from build123d import *

# Parameters (mm, degrees)
BOSS_EXTRUDE1_DEPTH       = 7
F_5_0MM_DOWEL_HOLE1_D     = 5
F_5_0MM_DOWEL_HOLE1_DEPTH = 7
SKETCH4_W                 = 66
SKETCH4_H                 = 37.5
BOSS_EXTRUDE2_DEPTH       = 13
SKETCH5_W                 = 65.8
SKETCH5_H                 = 37.3
BOSS_EXTRUDE3_DEPTH       = 22
FILLET1_R                 = 3
FILLET2_R                 = 2


with BuildPart() as part:
    # Sketch1 → Boss-Extrude1 (new body)
    with BuildSketch(Plane(origin=(0, 0, 0), x_dir=(1, 0, 0), z_dir=(0, 1, 0))):
        with BuildLine():
            Line((-41.327503189, 4.721250532), (-33, 15))
            Line((-33, 15), (-33, 26.5))
            Line((-33, 26.5), (33, 26.5))
            Line((33, 26.5), (33, 15))
            Line((33, 15), (41.327503189, 4.721250532))
            ThreePointArc((41.327503189, 4.721250532), (43, 0), (41.327503189, -4.721250532))
            Line((41.327503189, -4.721250532), (33, -15))
            Line((33, -15), (33, -26.5))
            Line((33, -26.5), (-33, -26.5))
            Line((-33, -26.5), (-33, -15))
            Line((-33, -15), (-41.327503189, -4.721250532))
            ThreePointArc((-41.327503189, -4.721250532), (-43, 0), (-41.327503189, 4.721250532))
        make_face()
    extrude(amount=BOSS_EXTRUDE1_DEPTH)

    # Ø5.0mm Dowel Hole1
    with Locations(Plane(origin=(0, 7, 0), x_dir=(1, 0, 0), z_dir=(0, 1, 0))):
        with Locations((-38.5, 0), (38.5, 0)):
            Hole(F_5_0MM_DOWEL_HOLE1_D / 2, depth=F_5_0MM_DOWEL_HOLE1_DEPTH)

    # Sketch4 → Boss-Extrude2 (add)
    with BuildSketch(Plane(origin=(0, 7, 0), x_dir=(1, 0, 0), z_dir=(0, 1, 0))):
        Rectangle(SKETCH4_W, SKETCH4_H)
    extrude(amount=BOSS_EXTRUDE2_DEPTH)

    # Sketch5 → Boss-Extrude3 (add)
    with BuildSketch(Plane(origin=(0, 20, 0), x_dir=(1, 0, 0), z_dir=(0, 1, 0))):
        Rectangle(SKETCH5_W, SKETCH5_H)
    extrude(amount=BOSS_EXTRUDE3_DEPTH)

    # Fillet1
    fillet1_edges = [part.edges().sort_by_distance(p)[0] for p in [
        (-33, 3.5, -26.5),
        (33, 3.5, -26.5),
        (33, 3.5, 26.5),
        (-33, 3.5, 26.5),
        (33, 13.5, 18.75),
        (33, 13.5, -18.75),
        (-33, 13.5, -18.75),
        (-33, 13.5, 18.75),
        (32.9, 31, 18.65),
        (32.9, 31, -18.65),
        (-32.9, 31, -18.65),
        (-32.9, 31, 18.65),
    ]]
    fillet(fillet1_edges, radius=FILLET1_R)

    # Fillet2
    fillet2_edges = [part.edges().sort_by_distance(p)[0] for p in [
        (32.9, 42, 0),
        (0, 42, 18.65),
        (0, 42, -18.65),
        (-32.9, 42, 0),
        (-32.021320344, 42, 17.771320344),
        (-32.021320344, 42, -17.771320344),
        (32.021320344, 42, -17.771320344),
        (32.021320344, 42, 17.771320344),
    ]]
    fillet(fillet2_edges, radius=FILLET2_R)


solid = part.part
Check sheet for the modelled part. Datum: model origin and axes. Units: mm. A direction names the side the tool comes from. Give positions to 0.01 mm unless a question says otherwise; leave off trailing zeros. Loops run counter-clockwise (first coordinate to the right, second up) from the corner with the lowest first, then second, coordinate; pieces in that order, holes last. Notation, with made-up numbers: M 53.5,61 L 110.5,61 A15 ccw 110.5,66 Z; hole C -17,9.25 d11. An arc over 180 degrees is marked long. Use a Markdown table: item, result. Add a question column.
Q1. Sectioned sample at D-D, the plane x = 20. Record the cut outline in (y, z).
Q2. Sectioned sample at A-A, the plane z = 0. Record the cut outline in (x, y), then the cut area to 3 significant figures.
Q3. Tool access check on faces 1 (the cylindrical face through (-32.14, 13.59, -17.85)), 2 (the cylindrical face through (32.04, 30.14, -17.75)), 3 (the flat face through (35.8, 7, -0.2)), 4 (the flat face through (-33, 10, 0)), 5 (the flat face through (0, 13, 18.75)). Record the directions out of +Z, -Z, +X, -X, +Y, -Y that give a thin tool (end or side, any length) a straight path to the whole face; none if there is none.
Q4. Scan lines: line 1 along Z through (x, y) = (-15, 11); line 2 along Y through (x, z) = (-12.5, -20); line 3 along X through (y, z) = (27.5, 10.5). Record each from-to range of solid material in increasing order. Write a range as [from, to].
Q5. Go/stop test with flat-tipped pins: pin 1 (10 mm diameter, centred on x = 8, y = 33.5, fed in from -Z); pin 2 (5 mm diameter, centred on x = 39.5, z = 6, fed in from +Y); pin 3 (6.5 mm diameter, centred on x = -4, y = 10.5, fed in from -Z). Record where each tip stops, or that it passes through.
Q6. Sectioned sample at B-B, the plane y = 37. Record the cut outline in (x, z), then the cut area to 3 significant figures.
Q7. Sectioned sample at C-C, the plane x = 37.5. Record the cut outline in (y, z).
Verdict:
| question | item | result |
|---|---|---|
| 1 | outline | M 0,-26.5 L 7,-26.5 L 7,-18.75 L 20,-18.75 L 20,-18.65 L 40,-18.65 A2 ccw 42,-16.65 L 42,16.65 A2 ccw 40,18.65 L 20,18.65 L 20,18.75 L 7,18.75 L 7,26.5 L 0,26.5 Z |
| 2 | outline | M -43,0 L -41,0 L -41,7 L -43,7 Z; M -36,0 L 36,0 L 36,7 L 33,7 L 33,20 L 32.9,20 L 32.9,40 A2 ccw 30.9,42 L -30.9,42 A2 ccw -32.9,40 L -32.9,20 L -33,20 L -33,7 L -36,7 Z; M 41,0 L 43,0 L 43,7 L 41,7 Z |
| 2 | area | 2,840 mm^2 |
| 3 | face 1 | -Z, -X, +Y |
| 3 | face 2 | -Z, +X, +Y |
| 3 | face 3 | +Z, -Z, +X, +Y |
| 3 | face 4 | -X, +Y |
| 3 | face 5 | +Z, +X, -X, +Y |
| 4 | line 1 | [-18.75, 18.75] |
| 4 | line 2 | [0, 7] |
| 4 | line 3 | [-32.9, 32.9] |
| 5 | pin 1 | z = -18.65 |
| 5 | pin 2 | y = 7 |
| 5 | pin 3 | z = -18.75 |
| 6 | outline | M -32.9,-15.65 A3 ccw -29.9,-18.65 L 29.9,-18.65 A3 ccw 32.9,-15.65 L 32.9,15.65 A3 ccw 29.9,18.65 L -29.9,18.65 A3 ccw -32.9,15.65 Z |
| 6 | area | 2,450 mm^2 |
| 7 | outline | M 0,-9.45 L 7,-9.45 L 7,-2.29 L 0,-2.29 Z; M 0,2.29 L 7,2.29 L 7,9.45 L 0,9.45 Z |
